```python
from build123d import *

# Parameters (mm, degrees)
SKETCH1_R             = 3.75
SKETCH1_R_2           = 1.5
BOSS_EXTRUDE1_DEPTH   = 5
BOSS_EXTRUDE1_2_DEPTH = 5
SKETCH2_R             = 1.5
BOSS_EXTRUDE2_DEPTH   = 1


with BuildPart() as part:
    # Sketch1 → Boss-Extrude1 (new body)
    with BuildSketch(Plane.XY):
        Circle(SKETCH1_R)
        Circle(SKETCH1_R_2, mode=Mode.SUBTRACT)
    extrude(amount=BOSS_EXTRUDE1_DEPTH)



with BuildPart() as body_2:
    # Sketch1 → Boss-Extrude1 2 (new body)
    with BuildSketch(Plane.XY):
        with Locations((13, 0)):
            Circle(SKETCH1_R)
        with Locations((13, 0)):
            Circle(SKETCH1_R_2, mode=Mode.SUBTRACT)
    extrude(amount=BOSS_EXTRUDE1_2_DEPTH)


with BuildPart() as part_1:
    add(part.part)

    add(body_2.part)  # Boss-Extrude2 merges body 2
    # Sketch2 → Boss-Extrude2 (add)
    with BuildSketch(Plane.XY.offset(5)):
        with BuildLine():
            ThreePointArc((0, 4.25), (-4.25, 0), (0, -4.25))
            add(Edge.make_bspline(
                [(0, -4.25), (2.386303511, -4.25), (6.863643386, -1.25), (9.886409718, -4.25), (13, -4.25)],
                knots=[0, 0, 0, 0, 0.5, 1, 1, 1, 1], degree=3))
            ThreePointArc((13, -4.25), (17.25, 0), (13, 4.25))
            add(Edge.make_bspline(
                [(0, 4.25), (2.386303511, 4.25), (6.863643386, 1.25), (9.886409718, 4.25), (13, 4.25)],
                knots=[0, 0, 0, 0, 0.5, 1, 1, 1, 1], degree=3))
        make_face()
        Circle(SKETCH2_R, mode=Mode.SUBTRACT)
        with Locations((13, 0)):
            Circle(SKETCH2_R, mode=Mode.SUBTRACT)
    boss_extrude2 = extrude(amount=BOSS_EXTRUDE2_DEPTH)

    # Mirror1: Boss-Extrude2 across plane
    add(boss_extrude2.mirror(Plane(origin=(0, 0, 2.5), x_dir=(1, 0, 0), z_dir=(0, 0, -1))))


solid = part_1.part
```
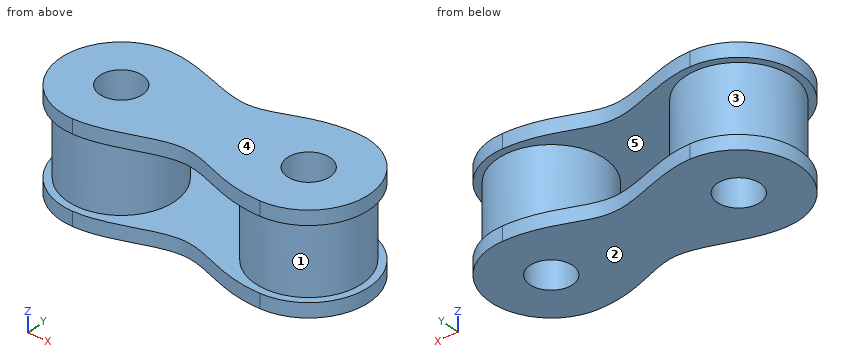
The model under review builds one solid part; all positions refer to its coordinate system, in mm. Face numbers are marked on the shaded views. A direction names the side the tool comes from. Coordinates: 2 decimals unless noted, no trailing zeros. Write each loop counter-clockwise with the first axis right and the second up, starting at its lowest first coordinate (ties: lowest second). Pieces come first, ordered by that corner, then holes. Notation, with made-up numbers: (25.25, -28.75) -> (48.25, -28.75) arc R16 ccw to (48.25, 2.25) -> close; hole circle Ø10 at (-12.75, 43.25). An arc over 180 degrees is marked (long way). One line per item, written item: value. Start each with the question number.
Q1. To check wall thickness, follow probe 1 along Z at (x, y) = (15.25, 3.5); probe 2 along X at (y, z) = (-1, 2.75); probe 3 along Y at (x, z) = (13, 1.25). State the ranges of each line that lie inside material, in increasing order.
Q2. Clearance check with flat-ended pins moving along their axes: P1, Ø4, axis at x = -1.5, z = 5, coming from the -Y side; P2, Ø2.5, axis at x = 0, y = 0, coming from the -Z side. State where each tip first meets the part, or that it passes through.
Q3. The part is to be moulded in two halves that separate along X. For the marked faces 1, 2 and 3, say which applies: +X half, -X half, draft (parallel to the pull), parting line (faces both ways), or undercut.
Q4. For the marked faces 4 and 5, list the 3-axis set-ups (+Z, -Z, +X, -X, +Y, -Y) from which the entire face can be reached by the end or side of a thin tool; tool diameter is ignored.
Q5. Add section C-C, the plane x = -1.25. Give the boundary of the cut face in (y, z), then the cut area to 3 significant figures.
Q6. Add section A-A, the plane y = 0. Give the boundary of the cut face in (x, z).
Q7. Add section B-B, the plane z = 1.5. Give the boundary of the cut face in (x, y), then the cut area to 3 significant figures.
Response:
1. probe 1: -1 to 0, 5 to 6
1. probe 2: -3.61 to -1.12, 1.12 to 3.61, 9.39 to 11.88, 14.12 to 16.61
1. probe 3: -3.75 to -1.5, 1.5 to 3.75
2. P1: y = -4.25
2. P2: through
3. face 1: undercut
3. face 2: draft
3. face 3: undercut
4. face 4: +Z, +X, -X, +Y, -Y
4. face 5: none
5. outline: (-4.06, -1) -> (-0.83, -1) -> (-0.83, 6) -> (-4.06, 6) -> (-4.06, 5) -> (-3.54, 5) -> (-3.54, 0) -> (-4.06, 0) -> close; (0.83, -1) -> (4.06, -1) -> (4.06, 0) -> (3.54, 0) -> (3.54, 5) -> (4.06, 5) -> (4.06, 6) -> (0.83, 6) -> close
5. area: 40.0 mm²
6. outline: (-4.25, -1) -> (-1.5, -1) -> (-1.5, 6) -> (-4.25, 6) -> (-4.25, 5) -> (-3.75, 5) -> (-3.75, 0) -> (-4.25, 0) -> close; (1.5, -1) -> (11.5, -1) -> (11.5, 6) -> (1.5, 6) -> close; (14.5, -1) -> (17.25, -1) -> (17.25, 0) -> (16.75, 0) -> (16.75, 5) -> (17.25, 5) -> (17.25, 6) -> (14.5, 6) -> close; hole (3.75, 0) -> (9.25, 0) -> (9.25, 5) -> (3.75, 5) -> close
7. outline: circle Ø7.5 at (0, 0); circle Ø7.5 at (13, 0); hole circle Ø3 at (0, 0); hole circle Ø3 at (13, 0)
7. area: 74.2 mm²
